from build123d import *

# Parameters (mm, degrees)
F0_W          = 1
F0_H          = 15
F0_W_2        = 15
F0_H_2        = 1
F1_DEPTH      = 1
F2_DEPTH      = 16
F3_W          = 2
F3_H          = 3
F3_W_2        = 3
F3_H_2        = 2
F4_DEPTH      = 3
F5_W          = 1
F5_H          = 1
F6_DEPTH      = 25
F7_DEPTH      = 2
F7_DEPTH_BACK = 15


with BuildPart() as f1:
    # F0 (on Top) → F1 (new body)
    with BuildSketch(Plane.XY):
        with Locations((8, 0)):
            Rectangle(F0_W, F0_H)
        with Locations((-16, -8)):
            Rectangle(F0_W_2, F0_H_2)
        with Locations((-16, 0)):
            Rectangle(F0_W_2, F0_H)
        with Locations((8, -16)):
            Rectangle(F0_W, F0_H)
        with Locations((0, -16)):
            Rectangle(F0_W_2, F0_H)
        with Locations((-8, -16)):
            Rectangle(F0_W, F0_H)
        with Locations((16, -16)):
            Rectangle(F0_W_2, F0_H)
        with Locations((-16, -16)):
            Rectangle(F0_W_2, F0_H)
        with Locations((16, 0)):
            Rectangle(F0_W_2, F0_H)
        with Locations((16, -8)):
            Rectangle(F0_W_2, F0_H_2)
        with Locations((0, -8)):
            Rectangle(F0_W_2, F0_H_2)
        with Locations((-8, 0)):
            Rectangle(F0_W, F0_H)
        Rectangle(F0_W_2, F0_H)
        with Locations((8, -8)):
            Rectangle(F0_W, F0_H_2)
        with Locations((-8, -8)):
            Rectangle(F0_W, F0_H_2)
        with Locations((-8, 8)):
            Rectangle(F0_W, F0_H_2)
        with Locations((-16, 8)):
            Rectangle(F0_W_2, F0_H_2)
        with Locations((8, 16)):
            Rectangle(F0_W, F0_H)
        with Locations((0, 16)):
            Rectangle(F0_W_2, F0_H)
        with Locations((-8, 16)):
            Rectangle(F0_W, F0_H)
        with Locations((16, 16)):
            Rectangle(F0_W_2, F0_H)
        with Locations((16, 8)):
            Rectangle(F0_W_2, F0_H_2)
        with Locations((-16, 16)):
            Rectangle(F0_W_2, F0_H)
        with Locations((8, 8)):
            Rectangle(F0_W, F0_H_2)
        with Locations((0, 8)):
            Rectangle(F0_W_2, F0_H_2)
    extrude(amount=-F1_DEPTH)

    # F0 (on Top) → F2 (join)
    with BuildSketch(Plane.XY):
        with Locations((-8, -8)):
            Rectangle(F0_W, F0_H_2)
        with Locations((8, -8)):
            Rectangle(F0_W, F0_H_2)
        with Locations((-8, 8)):
            Rectangle(F0_W, F0_H_2)
        with Locations((8, 8)):
            Rectangle(F0_W, F0_H_2)
        with Locations((16, 8)):
            Rectangle(F0_W_2, F0_H_2)
        with Locations((8, 16)):
            Rectangle(F0_W, F0_H)
        with Locations((-8, 16)):
            Rectangle(F0_W, F0_H)
        with Locations((0, 8)):
            Rectangle(F0_W_2, F0_H_2)
        with Locations((-16, 8)):
            Rectangle(F0_W_2, F0_H_2)
        with Locations((-8, 0)):
            Rectangle(F0_W, F0_H)
        with Locations((-16, -8)):
            Rectangle(F0_W_2, F0_H_2)
        with Locations((0, -8)):
            Rectangle(F0_W_2, F0_H_2)
        with Locations((16, -8)):
            Rectangle(F0_W_2, F0_H_2)
        with Locations((8, -16)):
            Rectangle(F0_W, F0_H)
        with Locations((-8, -16)):
            Rectangle(F0_W, F0_H)
        with Locations((8, 0)):
            Rectangle(F0_W, F0_H)
    extrude(amount=F2_DEPTH)

    # F3 (on face) → F4 (cut)
    with BuildSketch(Plane(origin=(0, 0, -1), x_dir=(1, 0, 0), z_dir=(0, 0, -1))):
        with BuildLine():
            Line((-7.5, 8.25), (-7.5, 7.5))
            Line((-7.5, 7.5), (-6.75, 7.5))
            ThreePointArc((-6.75, 7.5), (-6.9696699141, 8.0303300859), (-7.5, 8.25))
        make_face()
        with BuildLine():
            Line((-6.75, 7.5), (-7.5, 7.5))
            Line((-7.5, 7.5), (-7.5, 6.75))
            ThreePointArc((-7.5, 6.75), (-6.9696699141, 6.9696699141), (-6.75, 7.5))
        make_face()
        with BuildLine():
            Line((-7.5, 6.75), (-7.5, 7.5))
            Line((-7.5, 7.5), (-8.25, 7.5))
            ThreePointArc((-8.25, 7.5), (-8.0303300859, 6.9696699141), (-7.5, 6.75))
        make_face()
        with BuildLine():
            Line((-8.25, 7.5), (-7.5, 7.5))
            Line((-7.5, 7.5), (-7.5, 8.25))
            ThreePointArc((-7.5, 8.25), (-8.0303300859, 8.0303300859), (-8.25, 7.5))
        make_face()
        with BuildLine():
            Line((-1, 7.5), (-6.75, 7.5))
            ThreePointArc((-6.75, 7.5), (-6.9696699141, 6.9696699141), (-7.5, 6.75))
            Line((-7.5, 6.75), (-7.5, 1))
            Line((-7.5, 1), (-7.5, -1))
            Line((-7.5, -1), (-7.5, -6.75))
            ThreePointArc((-7.5, -6.75), (-6.9696699141, -6.9696699141), (-6.75, -7.5))
            Line((-6.75, -7.5), (-1, -7.5))
            Line((-1, -7.5), (1, -7.5))
            Line((1, -7.5), (6.75, -7.5))
            ThreePointArc((6.75, -7.5), (6.9696699141, -6.9696699141), (7.5, -6.75))
            Line((7.5, -6.75), (7.5, -1))
            Line((7.5, -1), (7.5, 1))
            Line((7.5, 1), (7.5, 6.75))
            ThreePointArc((7.5, 6.75), (6.9696699141, 6.9696699141), (6.75, 7.5))
            Line((6.75, 7.5), (1, 7.5))
            Line((1, 7.5), (-1, 7.5))
        make_face()
        with BuildLine():
            Line((-10.5, 7.5), (-8.25, 7.5))
            ThreePointArc((-8.25, 7.5), (-8.0303300859, 8.0303300859), (-7.5, 8.25))
            Line((-7.5, 8.25), (-7.5, 10.5))
            Line((-7.5, 10.5), (-10.5, 10.5))
            Line((-10.5, 10.5), (-10.5, 7.5))
        make_face()
        with Locations((0, 9)):
            Rectangle(F3_W, F3_H)
        with Locations((-9, 0)):
            Rectangle(F3_W_2, F3_H_2)
        with BuildLine():
            ThreePointArc((7.5, 8.25), (6.9696699141, 8.0303300859), (6.75, 7.5))
            Line((6.75, 7.5), (7.5, 7.5))
            Line((7.5, 7.5), (7.5, 8.25))
        make_face()
        with BuildLine():
            Line((7.5, 7.5), (6.75, 7.5))
            ThreePointArc((6.75, 7.5), (6.9696699141, 6.9696699141), (7.5, 6.75))
            Line((7.5, 6.75), (7.5, 7.5))
        make_face()
        with BuildLine():
            ThreePointArc((-6.75, -7.5), (-6.9696699141, -6.9696699141), (-7.5, -6.75))
            Line((-7.5, -6.75), (-7.5, -7.5))
            Line((-7.5, -7.5), (-6.75, -7.5))
        make_face()
        with BuildLine():
            Line((-7.5, -7.5), (-7.5, -6.75))
            ThreePointArc((-7.5, -6.75), (-8.0303300859, -6.9696699141), (-8.25, -7.5))
            Line((-8.25, -7.5), (-7.5, -7.5))
        make_face()
        with BuildLine():
            Line((8.25, 7.5), (7.5, 7.5))
            Line((7.5, 7.5), (7.5, 6.75))
            ThreePointArc((7.5, 6.75), (8.0303300859, 6.9696699141), (8.25, 7.5))
        make_face()
        with BuildLine():
            Line((7.5, 8.25), (7.5, 7.5))
            Line((7.5, 7.5), (8.25, 7.5))
            ThreePointArc((8.25, 7.5), (8.0303300859, 8.0303300859), (7.5, 8.25))
        make_face()
        with BuildLine():
            Line((7.5, 10.5), (7.5, 8.25))
            ThreePointArc((7.5, 8.25), (8.0303300859, 8.0303300859), (8.25, 7.5))
            Line((8.25, 7.5), (10.5, 7.5))
            Line((10.5, 7.5), (10.5, 10.5))
            Line((10.5, 10.5), (7.5, 10.5))
        make_face()
        with BuildLine():
            Line((-7.5, -8.25), (-7.5, -7.5))
            Line((-7.5, -7.5), (-8.25, -7.5))
            ThreePointArc((-8.25, -7.5), (-8.0303300859, -8.0303300859), (-7.5, -8.25))
        make_face()
        with BuildLine():
            Line((-6.75, -7.5), (-7.5, -7.5))
            Line((-7.5, -7.5), (-7.5, -8.25))
            ThreePointArc((-7.5, -8.25), (-6.9696699141, -8.0303300859), (-6.75, -7.5))
        make_face()
        with BuildLine():
            ThreePointArc((-7.5, -8.25), (-8.0303300859, -8.0303300859), (-8.25, -7.5))
            Line((-8.25, -7.5), (-10.5, -7.5))
            Line((-10.5, -7.5), (-10.5, -10.5))
            Line((-10.5, -10.5), (-7.5, -10.5))
            Line((-7.5, -10.5), (-7.5, -8.25))
        make_face()
        with Locations((9, 0)):
            Rectangle(F3_W_2, F3_H_2)
        with Locations((0, -9)):
            Rectangle(F3_W, F3_H)
        with BuildLine():
            ThreePointArc((8.25, -7.5), (8.0303300859, -6.9696699141), (7.5, -6.75))
            Line((7.5, -6.75), (7.5, -7.5))
            Line((7.5, -7.5), (8.25, -7.5))
        make_face()
        with BuildLine():
            Line((7.5, -7.5), (7.5, -6.75))
            ThreePointArc((7.5, -6.75), (6.9696699141, -6.9696699141), (6.75, -7.5))
            Line((6.75, -7.5), (7.5, -7.5))
        make_face()
        with BuildLine():
            Line((7.5, -7.5), (6.75, -7.5))
            ThreePointArc((6.75, -7.5), (6.9696699141, -8.0303300859), (7.5, -8.25))
            Line((7.5, -8.25), (7.5, -7.5))
        make_face()
        with BuildLine():
            Line((8.25, -7.5), (7.5, -7.5))
            Line((7.5, -7.5), (7.5, -8.25))
            ThreePointArc((7.5, -8.25), (8.0303300859, -8.0303300859), (8.25, -7.5))
        make_face()
        with BuildLine():
            Line((10.5, -7.5), (8.25, -7.5))
            ThreePointArc((8.25, -7.5), (8.0303300859, -8.0303300859), (7.5, -8.25))
            Line((7.5, -8.25), (7.5, -10.5))
            Line((7.5, -10.5), (10.5, -10.5))
            Line((10.5, -10.5), (10.5, -7.5))
        make_face()
    extrude(amount=-F4_DEPTH, mode=Mode.SUBTRACT)

    # F5 (on face) → F6 (cut)
    with BuildSketch(Plane.XY.offset(16)):
        with Locations((-8, 23)):
            Rectangle(F5_W, F5_H)
        with Locations((-23, 8)):
            Rectangle(F5_W, F5_H)
        with Locations((8, 23)):
            Rectangle(F5_W, F5_H)
        with Locations((23, 8)):
            Rectangle(F5_W, F5_H)
        with Locations((23, -8)):
            Rectangle(F5_W, F5_H)
        with Locations((8, -23)):
            Rectangle(F5_W, F5_H)
        with Locations((-8, -23)):
            Rectangle(F5_W, F5_H)
        with Locations((-23, -8)):
            Rectangle(F5_W, F5_H)
    extrude(amount=-F6_DEPTH, mode=Mode.SUBTRACT)

    # F5 (on face) → F7 (join, two sides)
    with BuildSketch(Plane.XY.offset(16)) as f7_sk:
        with Locations((-8, 23)):
            Rectangle(F5_W, F5_H)
        with Locations((-23, 8)):
            Rectangle(F5_W, F5_H)
        with Locations((8, 23)):
            Rectangle(F5_W, F5_H)
        with Locations((23, 8)):
            Rectangle(F5_W, F5_H)
        with Locations((23, -8)):
            Rectangle(F5_W, F5_H)
        with Locations((8, -23)):
            Rectangle(F5_W, F5_H)
        with Locations((-8, -23)):
            Rectangle(F5_W, F5_H)
        with Locations((-23, -8)):
            Rectangle(F5_W, F5_H)
    extrude(amount=F7_DEPTH)
    extrude(f7_sk.sketch, amount=-F7_DEPTH_BACK)


solid = f1.part
Geometry: final body of the model. Coordinates: model frame, mm. A direction names the side the tool comes from. Give positions to 0.01 mm unless a question says otherwise; leave off trailing zeros. Loops run counter-clockwise (first coordinate to the right, second up) from the corner with the lowest first, then second, coordinate; pieces in that order, holes last. Notation, with made-up numbers: (-32, 0.5) - (19, 0.5) arc R9 cw to (19, 10.5) - close; hole circle Ø10 at (76, -7.5). An arc over 180 degrees is marked (long way). Answer as CSV lines item,"result". Start each with the question number.
1. Section D-D, the plane x = 19. Return loops of the section in (y, z).
2. Pin query (flat end, axial travel): P1, Ø4.5, axis at y = 17.5, z = 5.5, coming from the +X side; P2, Ø10, axis at x = 14, z = 5.5, coming from the +Y side; P3, Ø8, axis at y = -2, z = 7.5, coming from the -X side. Return the tip coordinate at first contact, or that it passes through.
3. Ray query, L1, parallel to Y at x = 14, z = 9.5; L2, parallel to Z at x = -15, y = 2. Return the intervals inside material, ascending.
4. Section A-A, the plane x = -2. Return loops of the section in (y, z), plus the area to 3 significant figures.
5. Reachability of faces 5 (the face through (-7.5, 16, 9)), 6 (the face through (7.5, 0, 7)), 7 (the face through (-1, 8, 0)) from +Z, -Z, +X, -X, +Y, -Y: full face, straight path, thin tool, end or side. Return the list, or none.
6. Draft query along Y for faces 1 (the face through (9.1, -7.5, -0.2)), 2 (the face through (-16, -8.5, 9)), 3 (the face through (-16, 8.5, 9)), 4 (the face through (-16, 16, 0)). Return one class per face: released by +Y, released by -Y, zero draft, split by the parting line, or undercut.
Answers:
1,outline,"(-23.5, -1) - (23.5, -1) - (23.5, 0) - (8.5, 0) - (8.5, 16) - (7.5, 16) - (7.5, 0) - (-7.5, 0) - (-7.5, 16) - (-8.5, 16) - (-8.5, 0) - (-23.5, 0) - close"
2,P1,"stops at x = 8.5"
2,P2,"stops at y = 8.5"
2,P3,"stops at x = -8.5"
3,L1,"y = -8.5 to -7.5, 7.5 to 8.5"
3,L2,"z = -1 to 0"
4,outline,"(-23.5, -1) - (-7.5, -1) - (-7.5, 16) - (-8.5, 16) - (-8.5, 0) - (-23.5, 0) - close; (7.5, -1) - (23.5, -1) - (23.5, 0) - (8.5, 0) - (8.5, 16) - (7.5, 16) - close"
4,area,"64.0 mm2"
5,face 5,"+Z, +Y"
5,face 6,"+Z, -Z"
5,face 7,"-Z"
6,face 1,"undercut"
6,face 2,"released by -Y"
6,face 3,"released by +Y"
6,face 4,"zero draft"
